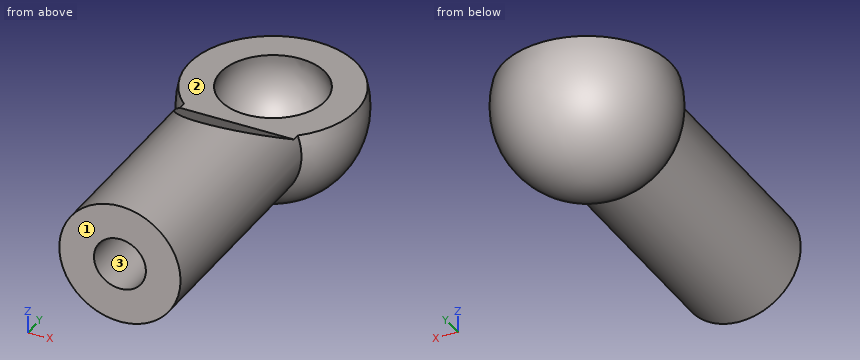
```python
from build123d import *

# Parameters (mm, degrees)
F2_R          = 3.5
F3_DEPTH      = 17
F7_DEPTH      = 6
F7_DEPTH_BACK = 6
F8_R          = 1.5
F9_DEPTH      = 8


with BuildPart() as f1:
    # F0 (on Right) → F1 (revolve)
    with BuildSketch(Plane.YZ):
        with BuildLine():
            Line((0, 5), (0, -5))
            ThreePointArc((0, -5), (5, 0), (0, 5))
        make_face()
    revolve(axis=Axis((0, 0, 0), (0, 0, -1)))

    # F2 (on Front) → F3 (join)
    with BuildSketch(Plane.XZ):
        Circle(F2_R)
    extrude(amount=F3_DEPTH)

    # F4 (on Right) → F5 (revolve, cut)
    with BuildSketch(Plane.YZ):
        with BuildLine():
            Line((0, 3.25), (0, -3.25))
            ThreePointArc((0, -3.25), (3.25, 0), (0, 3.25))
        make_face()
    revolve(axis=Axis((0, 0, 0), (0, 0, -1)), mode=Mode.SUBTRACT)

    # F6 (on Right) → F7 (cut, two sides)
    with BuildSketch(Plane.YZ) as f7_sk:
        Polygon((-4, 1.2), (5.5, 1.2), (5.5, 5.2), (-10.9282032303, 5.2), align=None)
    extrude(amount=-F7_DEPTH, mode=Mode.SUBTRACT)
    extrude(f7_sk.sketch, amount=F7_DEPTH_BACK, mode=Mode.SUBTRACT)

    # F8 (on face) → F9 (cut)
    with BuildSketch(Plane.XZ.offset(17)):
        Circle(F8_R)
    extrude(amount=-F9_DEPTH, mode=Mode.SUBTRACT)


solid = f1.part
```
Check sheet for the modelled part. Datum: model origin and axes. Units: mm. Face numbers are marked on the shaded views. A direction names the side the tool comes from. Give positions to 0.01 mm unless a question says otherwise; leave off trailing zeros. Order: outer loops, then holes, each group sorted by start corner. A loop starts at its lowest first (then second) coordinate and runs counter-clockwise, first axis right, second up. Notation, with made-up numbers: M 11,-39.75 L 30,-39.75 A16 ccw 30,-34.75 Z; hole C 63.25,62.5 d3. An arc over 180 degrees is marked long. Answer in a Markdown table with one row per item. Add a question column.
Q1. Sectioned sample at C-C, the plane z = -2.25. Record the boundary of the cut face in (x, y), and give its area (3 significant figures).
Q2. Gauge pin test, flat ends, axial feed: pin 1 Ø1 at (x, y) = (3, -12.5) entering from -Z; pin 2 Ø4 at (y, z) = (-11, -1.5) entering from -X; pin 3 Ø4 at (y, z) = (-10.5, -3.5) entering from -X. Record the tip position at first contact, or that the pin passes through.
Q3. Access from +Z, -Z, +X, -X, +Y, -Y to the whole of each face (thin tool, end or side, straight path). Record for the marked faces 1, 2 and 3.
Q4. Sectioned sample at B-B, the plane x = -0.25. Record the boundary of the cut face in (y, z).
Q5. Sectioned sample at A-A, the plane z = 0. Record the boundary of the cut face in (x, y).
Q6. Thickness scan on L1, parallel to Y at x = 0, z = 0; L2, parallel to Z at x = 0, y = -14; L3, parallel to X at y = 2.5, z = 0.5. Record the ranges inside material, lowest first.
Q7. Sectioned sample at D-D, the plane y = -2.25. Record the boundary of the cut face in (x, z), and give its area (3 significant figures).
Verdict:
| question | item | result |
|---|---|---|
| 1 | outline | M -2.68,-17 L 2.68,-17 L 2.68,-3.57 A4.47 ccw long -2.68,-3.57 Z; hole C 0,0 d4.69 |
| 1 | area | 114 mm² |
| 2 | pin 1 | z = -2.45 |
| 2 | pin 2 | x = -3.5 |
| 2 | pin 3 | x = -3.16 |
| 3 | face 1 | +Z, -Z, +X, -X, -Y |
| 3 | face 2 | +Z, +X, -X, +Y |
| 3 | face 3 | -Y |
| 4 | outline | M -17,-3.49 L -3.57,-3.49 A4.99 ccw 4.85,1.2 L 3.01,1.2 A3.24 cw long -3.01,1.2 L -4,1.2 L -7.97,3.49 L -17,3.49 L -17,1.48 L -9,1.48 L -9,-1.48 L -17,-1.48 Z |
| 5 | outline | M -3.5,-17 L -1.5,-17 L -1.5,-9 L 1.5,-9 L 1.5,-17 L 3.5,-17 L 3.5,-3.57 A5 ccw long -3.5,-3.57 Z; hole C 0,0 d6.5 |
| 6 | L1 | -9 to -3.25, 3.25 to 5 |
| 6 | L2 | -3.5 to -1.5, 1.5 to 3.5 |
| 6 | L3 | -4.3 to -2.02, 2.02 to 4.3 |
| 7 | outline | M -4.3,1.2 A4.47 ccw long 4.3,1.2 L 2.01,1.2 A2.35 cw long -2.01,1.2 Z |
| 7 | area | 27.9 mm² |
